Autodesk Inventor part; units mm, degrees
ref_plane "YZ Plane" through (0, 0, 0) normal (1, 0, 0) x (0, 1, 0)
ref_plane "XZ Plane" through (0, 0, 0) normal (0, 1, 0) x (-1, 0, 0)
ref_plane "XY Plane" through (0, 0, 0) normal (0, 0, 1) x (1, 0, 0)
sketch "Sketch1" plane through (0, 0, 0) normal (0, 0, 1) x (1, 0, 0)
  line L0 (-5, 0) -> (5, 0)
  line L1 (-5, 0) -> (-5, 10)
  line L2 (-5, 10) -> (-3, 12)
  line L3 (-3, 12) -> (3, 12)
  line L4 (3, 12) -> (5, 10)
  line L5 (5, 10) -> (5, 0)
  point P0 (0, 0)
  point P1 (0, 0)
  point P2 (0, 12)
  dimension "d0" = 10
  dimension "d1" = 24
  dimension "d2" = 6
  dimension "d3" = 20
revolve "Revolution1" add sketch "Sketch1" angle 360 about axis through (-5, 0, 0) along (1, 0, 0)
sketch "Sketch2" plane through (5, 0, 0) normal (1, 0, 0) x (0, 0, -1)
  circle A0 centre (0, 0) radius 2.5
  dimension "d5" = 5
extrude "Extrusion1" cut sketch "Sketch2" against normal through all
sketch "Sketch3" plane through (5, 0, 0) normal (1, 0, 0) x (0, 0, -1)
  circle A0 centre (0, 0) radius 4
  circle A1 centre (0, 0) radius 2.5
  dimension "d8" = 8
extrude "Extrusion2" add sketch "Sketch3" along normal blind 6
sketch "Sketch4" plane through (-5, 0, 0) normal (-1, 0, 0) x (0, 0, 1)
  circle A0 centre (0, 0) radius 2.5
  circle A1 centre (0, 0) radius 4
  dimension "d11" = 8
extrude "Extrusion3" add sketch "Sketch4" along normal blind 6
properties part number "wheel"
Here's how the part is built. I have some questions about the finished solid (model axes, mm). A direction names the side the tool comes from. Coordinates: 2 decimals unless noted, no trailing zeros. Write each loop counter-clockwise with the first axis right and the second up, starting at its lowest first coordinate (ties: lowest second). Pieces come first, ordered by that corner, then holes.
Item 1: I want a section at B-B on x = -5.5. Write out the boundary of the cut face in (y, z), and give its area (3 significant figures).
Item 2: On a 3-axis mill with a long thin cutter (end or side, diameter ignored), from which of +Z, -Z, +X, -X, +Y, -Y can I reach the whole of each face in a straight line? I mean faces 1 (the flat face through (-5, 4.3, 0.1)), 2 (the flat face through (11, 2, -2)), 3 (the cylindrical face through (7.958, 3.905, 0.867)). Say none if no direction works.
Item 3: If I drill on line 1 (Z direction, x = -0.5, y = 0); line 2 (Y direction, x = -6, z = 0); line 3 (Y direction, x = 4, z = 0), over which ranges is the centre line in solid material (lowest first)?
Item 4: Will these pins go through, and if not, where does the flat tip stop? pin 1 (8 mm diameter, centred on x = -0.5, z = -8, fed in from -Y); pin 2 (3 mm diameter, centred on x = 8.5, z = -6.5, fed in from -Y); pin 3 (5 mm diameter, centred on y = -7, z = -5.5, fed in from +X); pin 4 (1.5 mm diameter, centred on x = -4.5, z = -6, fed in from +Y).
Item 5: If we mould it in two halves opening along Y, with no side actions, what happens to faces 4 (the cylindrical face through (0.154, 2.495, -0.165)), 5 (the cylindrical face through (-7.958, 3.905, -0.867)), 6 (the flat face through (5, 4.3, 0.1))? For each: +Y half, -Y half, draft (parallel to the pull), parting line (faces both ways), or undercut.
Item 6: I want a section at A-A on y = 0. Write out the boundary of the cut face in (x, z), and give its area (3 significant figures).
Findings below:
1. outline: circle Ø8 at (0, 0); hole circle Ø5 at (0, 0)
1. area: 30.6 mm2
2. face 1: -X
2. face 2: +Z, -Z, +X, +Y, -Y
2. face 3: +X
3. line 1: z = -12 to -2.5, 2.5 to 12
3. line 2: y = -4 to -2.5, 2.5 to 4
3. line 3: y = -11 to -2.5, 2.5 to 11
4. pin 1: stops at y = -11.31
4. pin 2: passes through
4. pin 3: stops at x = 5
4. pin 4: stops at y = 9.63
5. face 4: undercut
5. face 5: parting line
5. face 6: draft
6. outline: (-11, -4) - (-5, -4) - (-5, -10) - (-3, -12) - (3, -12) - (5, -10) - (5, -4) - (11, -4) - (11, -2.5) - (-11, -2.5) - close; (-11, 2.5) - (11, 2.5) - (11, 4) - (5, 4) - (5, 10) - (3, 12) - (-3, 12) - (-5, 10) - (-5, 4) - (-11, 4) - close
6. area: 218 mm2
